```python
from build123d import *

# Parameters (mm, degrees)
SKETCH1_R      = 1.3
EXTRUDE1_DEPTH = 0.35


with BuildPart() as part:
    # Sketch1 → Extrude1 (new body)
    with BuildSketch(Plane(origin=(0, 0, 0), x_dir=(0, 0, -1), z_dir=(1, 0, 0))):
        with BuildLine():
            Line((-12.885760186, 5.95357069), (-13.381095839, 6.907130708))
            ThreePointArc((-13.381095839, 6.907130708), (-13.603001468, 7.943369547), (-13.264308138, 8.947520865))
            ThreePointArc((-13.264308138, 8.947520865), (0, 16), (13.264308138, 8.947520865))
            ThreePointArc((13.264308138, 8.947520865), (13.603001468, 7.943369547), (13.381095839, 6.907130708))
            Line((13.381095839, 6.907130708), (12.885760186, 5.95357069))
            ThreePointArc((12.885760186, 5.95357069), (12.66609567, 5.17996722), (12.768897836, 4.382379268))
            ThreePointArc((12.768897836, 4.382379268), (11.972673932, -6.2373936), (3.725896212, -12.97565788))
            ThreePointArc((3.725896212, -12.97565788), (2.889265769, -13.458620697), (2.376600464, -14.277386759))
            ThreePointArc((2.376600464, -14.277386759), (0, -16.001648251), (-2.376600464, -14.277386759))
            ThreePointArc((-2.376600464, -14.277386759), (-2.889265769, -13.458620697), (-3.725896212, -12.97565788))
            ThreePointArc((-3.725896212, -12.97565788), (-11.972673932, -6.2373936), (-12.768897836, 4.382379268))
            ThreePointArc((-12.768897836, 4.382379268), (-12.66609567, 5.17996722), (-12.885760186, 5.95357069))
        make_face()
        with Locations((11, 7.829080757)):
            Circle(SKETCH1_R, mode=Mode.SUBTRACT)
        with Locations((-11, 7.829080757)):
            Circle(SKETCH1_R, mode=Mode.SUBTRACT)
        with Locations((0, -13.501648251)):
            Circle(SKETCH1_R, mode=Mode.SUBTRACT)
        with BuildLine():
            Line((-5, 13.25), (5, 13.25))
            ThreePointArc((5, 13.25), (5.707106781, 12.957106781), (6, 12.25))
            Line((6, 12.25), (6, 10.656570743))
            ThreePointArc((6, 10.656570743), (6.119937614, 10.181712663), (6.450980392, 9.820761273))
            ThreePointArc((6.450980392, 9.820761273), (0, -11.75), (-6.450980392, 9.820761273))
            ThreePointArc((-6.450980392, 9.820761273), (-6.119937614, 10.181712663), (-6, 10.656570743))
            Line((-6, 10.656570743), (-6, 12.25))
            ThreePointArc((-6, 12.25), (-5.707106781, 12.957106781), (-5, 13.25))
        make_face(mode=Mode.SUBTRACT)
    extrude(amount=EXTRUDE1_DEPTH)


solid = part.part
```
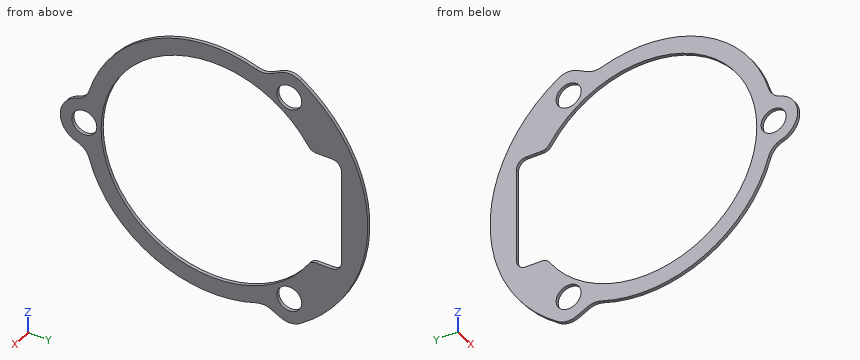
Verification items for the finished model (mm, model axes). Round coordinates to 2 decimals unless told otherwise and drop trailing zeros. Write each loop counter-clockwise with the first axis right and the second up, starting at its lowest first coordinate (ties: lowest second). Pieces come first, ordered by that corner, then holes. Notation, with made-up numbers: (27.5, -34) - (53.5, -34) arc R11 cw to (53.5, -15) - close; hole circle Ø3 at (86.25, -17). An arc over 180 degrees is marked (long way). Answer as a JSON object with one key per item and string values. Group by question number.
Q1. Section check A-A, the plane y = 0. Enter the section's corners in (x, z).
Q2. Section check B-B, the plane z = 0. Enter the section's corners in (x, y).
Q3. Section check D-D, the plane y = -8.5. Enter the section's corners in (x, z), plus the area to 3 significant figures.
Q4. Thickness scan on line 1 (Z direction, x = 0.2, y = 0); line 2 (Y direction, x = 0.25, z = -8.5); line 3 (Z direction, x = 0.1, y = -6). Record the ranges inside material, lowest first.
Q5. Section check C-C, the plane x = 0.25. Enter the section's corners in (y, z), plus the area to 3 significant figures.
Found:
{
 "1": {"outline": "(0, -13.5) - (0.35, -13.5) - (0.35, -11.75) - (0, -11.75) - close; (0, 11.75) - (0.35, 11.75) - (0.35, 13.5) - (0, 13.5) - close"},
 "2": {"outline": "(0, -16) - (0.35, -16) - (0.35, -14.8) - (0, -14.8) - close; (0, -12.2) - (0.35, -12.2) - (0.35, -11.75) - (0, -11.75) - close; (0, 13.25) - (0.35, 13.25) - (0.35, 16) - (0, 16) - close"},
 "3": {"outline": "(0, -10.49) - (0.35, -10.49) - (0.35, -8.11) - (0, -8.11) - close; (0, 8.11) - (0.35, 8.11) - (0.35, 10.49) - (0, 10.49) - close", "area": "1.66 mm^2"},
 "4": {"line 1": "z = -13.5 to -11.75, 11.75 to 13.5", "line 2": "y = -10.49 to -8.11, 8.11 to 13.56", "line 3": "z = -12.09 to -10.1, 10.1 to 12.09"},
 "5": {"outline": "(-14.28, -2.38) arc R2 cw to (-12.98, -3.73) arc R13.5 ccw to (4.38, -12.77) arc R2 cw to (5.95, -12.89) - (6.91, -13.38) arc R2 ccw to (8.95, -13.26) arc R16 ccw to (8.95, 13.26) arc R2 ccw to (6.91, 13.38) - (5.95, 12.89) arc R2 cw to (4.38, 12.77) arc R13.5 ccw to (-12.98, 3.73) arc R2 cw to (-14.28, 2.38) arc R2.5 ccw to start; hole circle Ø2.6 at (-13.5, 0); hole circle Ø2.6 at (7.83, -11); hole circle Ø2.6 at (7.83, 11); hole (9.82, -6.45) arc R1 cw to (10.66, -6) - (12.25, -6) arc R1 ccw to (13.25, -5) - (13.25, 5) arc R1 ccw to (12.25, 6) - (10.66, 6) arc R1 cw to (9.82, 6.45) arc R11.75 ccw (long way) to start", "area": "191 mm^2"}
}
